from build123d import *

# Parameters (mm, degrees)
SKETCH_1_R          = 5
SKETCH_1_R_2        = 3
EXTRUDE_1_DEPTH     = 4
SKETCH_2_R          = 5.75
EXTRUDE_2_DEPTH     = 0.9
SKETCH_3_R          = 3
CUT_EXTRUDE_2_DEPTH = 9.9
SKETCH_2_2_R        = 5.75
EXTRUDE_3_DEPTH     = 1
SKETCH_3_2_R        = 3
CUT_EXTRUDE_3_DEPTH = 7


with BuildPart() as part:
    # 草图1 → 凸台-拉伸1 (new body)
    with BuildSketch(Plane.XY):
        Circle(SKETCH_1_R)
        Circle(SKETCH_1_R_2, mode=Mode.SUBTRACT)
    extrude(amount=EXTRUDE_1_DEPTH)

    # 草图2 → 凸台-拉伸2 (add)
    with BuildSketch(Plane.XY):
        Circle(SKETCH_2_R)
    extrude(amount=EXTRUDE_2_DEPTH)

    # 草图3 → 切除-拉伸2 (cut)
    with BuildSketch(Plane.XY):
        Circle(SKETCH_3_R)
    extrude(amount=CUT_EXTRUDE_2_DEPTH, mode=Mode.SUBTRACT)

    # 草图2<2> → 凸台-拉伸3 (add)
    with BuildSketch(Plane.XY):
        Circle(SKETCH_2_2_R)
    extrude(amount=EXTRUDE_3_DEPTH)

    # 草图3<2> → 切除-拉伸3 (cut)
    with BuildSketch(Plane.XY):
        Circle(SKETCH_3_2_R)
    extrude(amount=CUT_EXTRUDE_3_DEPTH, mode=Mode.SUBTRACT)


solid = part.part
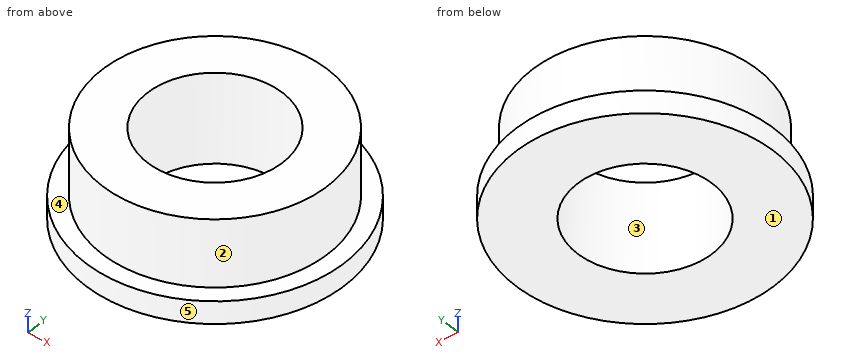
Work out the finished part from the listing and answer in its coordinate system (mm). Face numbers are marked on the shaded views. A direction names the side the tool comes from. Coordinates: 2 decimals unless noted, no trailing zeros. Write each loop counter-clockwise with the first axis right and the second up, starting at its lowest first coordinate (ties: lowest second). Pieces come first, ordered by that corner, then holes. Notation, with made-up numbers: M 31,25 L 52,25 A10 ccw 52,40 Z; hole C 14.25,42.5 d4. An arc over 180 degrees is marked long. Use one line per item in the form item = value. Start each with the question number.
1. The part is cut by section D-D (x = 3.5). Give the vertices of the cut face in (y, z), plus the area to 3 significant figures.
2. The part is cut by section C-C (z = 2.55). Give the vertices of the cut face in (x, y), plus the area to 3 significant figures.
3. A tool of negligible diameter and unlimited length cuts with its end or side. For the marked faces 1 and 2, from which of +Z, -Z, +X, -X, +Y, -Y can it reach the whole face along a straight path? Write none if from no direction.
4. Each of these flat-tipped pins is pushed along its axis until it touches: P1, Ø6, axis at x = 0, y = -0.5, coming from the +Z side; P2, Ø3.5, axis at x = 0, y = 0, coming from the -Z side; P3, Ø1.5, axis at x = -2, z = 3, coming from the -Y side; P4, Ø1.5, axis at y = -1, z = 2.5, coming from the +X side. Where does it stop, or does it pass through?
5. The mould has two halves that part along Y. Classify the marked faces 3, 4 and 5: released by +Y, released by -Y, zero draft, split by the parting line, or undercut.
6. Straight lines are drawn through the part: probe 1 along Y at (x, z) = (0, 3.1); probe 2 along X at (y, z) = (1.5, 3.35); probe 3 along Y at (x, z) = (-2.25, 2.8). For each, find the intervals that lie inside material, in ascending order. Write a range as from..to.
7. The part is cut by section A-A (x = 0). Give the vertices of the cut face in (y, z).
Evaluation:
q1.outline = M -4.56,0 L 4.56,0 L 4.56,1 L 3.57,1 L 3.57,4 L -3.57,4 L -3.57,1 L -4.56,1 Z
q1.area = 30.5 mm^2
q2.outline = C 0,0 d10; hole C 0,0 d6
q2.area = 50.3 mm^2
q3.face_1 = -Z, +X, -X, +Y, -Y
q3.face_2 = +Z
q4.P1 = 4
q4.P2 = through
q4.P3 = -4.84
q4.P4 = 4.99
q5.face_3 = undercut
q5.face_4 = zero draft
q5.face_5 = split by the parting line
q6.probe_1 = -5..-3, 3..5
q6.probe_2 = -4.77..-2.6, 2.6..4.77
q6.probe_3 = -4.47..-1.98, 1.98..4.47
q7.outline = M -5.75,0 L -3,0 L -3,4 L -5,4 L -5,1 L -5.75,1 Z; M 3,0 L 5.75,0 L 5.75,1 L 5,1 L 5,4 L 3,4 Z
